```python
from build123d import *

# Parameters (mm, degrees)
F0_R     = 11
F0_R_2   = 6
F1_DEPTH = 2
F0_R_3   = 3.895
F2_DEPTH = 3
F3_DEPTH = 6.5
F4_R     = 0.5
F5_R     = 0.5


with BuildPart() as f1:
    # F0 (on Top) → F1 (new body)
    with BuildSketch(Plane.XY):
        Circle(F0_R)
        Circle(F0_R_2, mode=Mode.SUBTRACT)
    extrude(amount=F1_DEPTH)

    # F0 (on Top) → F2 (join)
    with BuildSketch(Plane.XY):
        Circle(F0_R_2)
        Circle(F0_R_3, mode=Mode.SUBTRACT)
    extrude(amount=F2_DEPTH)

    # F0 (on Top) → F3 (join)
    with BuildSketch(Plane.XY):
        Circle(F0_R_3)
    extrude(amount=F3_DEPTH)

    # F4
    f4_edges = [f1.edges().sort_by_distance(p)[0] for p in [
        (-3.895, 0, 6.5),
    ]]
    fillet(f4_edges, radius=F4_R)

    # F5
    f5_edges = [f1.edges().sort_by_distance(p)[0] for p in [
        (-11, 0, 0),
        (-11, 0, 2),
    ]]
    fillet(f5_edges, radius=F5_R)


solid = f1.part
```
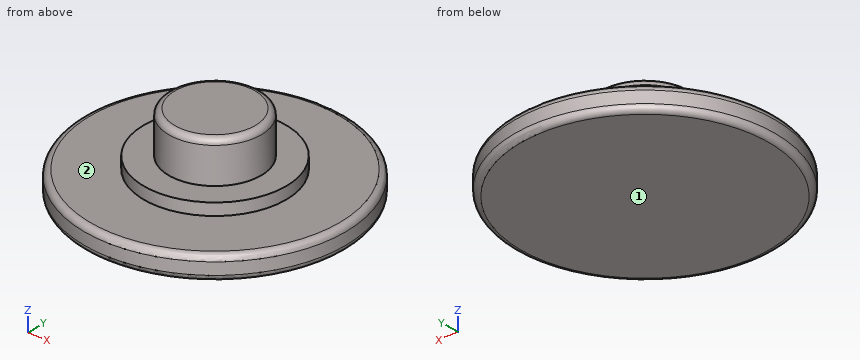
The model under review builds one solid part; all positions refer to its coordinate system, in mm. Face numbers are marked on the shaded views. A direction names the side the tool comes from. Round coordinates to 2 decimals unless told otherwise and drop trailing zeros. Order: outer loops, then holes, each group sorted by start corner. A loop starts at its lowest first (then second) coordinate and runs counter-clockwise, first axis right, second up. Notation, with made-up numbers: (49, 52) -> (69, 52) arc R21 cw to (69, 75) -> close; hole circle Ø4 at (46.25, 23). An arc over 180 degrees is marked (long way). One line per item, written item: value. Start each with the question number.
Q1. Machinability: for the marked faces 1 and 2, which of the approach directions +Z, -Z, +X, -X, +Y, -Y give a long, thin tool a straight path to every point of the face, cutting with its end or side? Answer none if there is none.
Q2. Take a section at C-C (z = 5). Write out the cut boundary in (x, y) (3 decimals).
Q3. Take a section at A-A (x = 0). Write out the cut boundary in (y, z) (3 decimals), and give its area (3 significant figures).
Q4. Wall thickness on line 1 (Z direction, x = 9.75, y = 1.75); line 2 (Z direction, x = 1, y = -5); line 3 (X direction, y = 2, z = 0.5): over which ranges is each line inside the solid? List them lowest first.
Q5. Clearance check with a flat-ended pin moving along its axis: pin 1 Ø1.5 at (x, y) = (-2.5, -4.5) entering from +Z. State where the tip first meets the part, or that it passes through.
Reported:
1. face 1: -Z, +X, -X, +Y, -Y
1. face 2: +Z
2. outline: circle Ø7.79 at (0, 0)
3. outline: (-11, 0.5) arc R0.5 ccw to (-10.5, 0) -> (10.5, 0) arc R0.5 ccw to (11, 0.5) -> (11, 1.5) arc R0.5 ccw to (10.5, 2) -> (6, 2) -> (6, 3) -> (3.895, 3) -> (3.895, 6) arc R0.5 ccw to (3.395, 6.5) -> (-3.395, 6.5) arc R0.5 ccw to (-3.895, 6) -> (-3.895, 3) -> (-6, 3) -> (-6, 2) -> (-10.5, 2) arc R0.5 ccw to (-11, 1.5) -> close
3. area: 82.9 mm2
4. line 1: z = 0 to 2
4. line 2: z = 0 to 3
4. line 3: x = -10.82 to 10.82
5. pin 1: stops at z = 3
